Design review of the part built by this model. Coordinates are the model's own, in mm. A direction names the side the tool comes from. Coordinates: 2 decimals unless noted, no trailing zeros. Write each loop counter-clockwise with the first axis right and the second up, starting at its lowest first coordinate (ties: lowest second). Pieces come first, ordered by that corner, then holes.
Q1. Add section D-D, the plane x = -5.5. Give the boundary of the cut face in (y, z).
Q2. To check wall thickness, follow probe 1 along Y at (x, z) = (20, 3); probe 2 along X at (y, z) = (4, -53.5); probe 3 along Z at (x, y) = (36.5, 8). State the ranges of each line that lie inside material, in increasing order.
Q3. Add section C-C, the plane x = -16.5. Give the boundary of the cut face in (y, z).
Q4. Clearance check with flat-ended pins moving along their axes: pin 1 Ø2.5 at (x, y) = (-34.5, 29) entering from +Z; pin 2 Ø0.9 at (x, y) = (-35, 29) entering from -Z; pin 3 Ø12 at (x, z) = (-25.5, 26.5) entering from +Y. State where each tip first meets the part, or that it passes through.
Q5. The part is to be moulded in two halves that separate along X. For faces 1 (the face through (2, 0, 1)), 2 (the face through (38, 2, 73)), 3 (the face through (24.847, 12.86, 87.158)), say which applies: +X half, -X half, draft (parallel to the pull), parting line (faces both ways), or undercut.
Q6. Machinability: for faces 4 (the face through (-24.451, 12.86, 87.316)), 5 (the face through (-38, 9, -80.5)), 6 (the face through (-41.019, 17, -1)), 7 (the face through (38, 2, -73)), which of the approach directions +Z, -Z, +X, -X, +Y, -Y give a long, thin tool a straight path to every point of the face, cutting with its end or side? Answer none if there is none.
Q7. Add section B-B, the plane y = 15.5. Give the boundary of the cut face in (x, z).
Autodesk Inventor part; units mm, degrees
ref_plane "YZ Plane" through (0, 0, 0) normal (1, 0, 0) x (0, 1, 0)
ref_plane "XZ Plane" through (0, 0, 0) normal (0, 1, 0) x (-1, 0, 0)
ref_plane "XY Plane" through (0, 0, 0) normal (0, 0, 1) x (1, 0, 0)
sketch "Sketch1" plane through (0, 0, 0) normal (0, 1, 0) x (-1, 0, 0)
  line L0 (38, 68) -> (38, -68)
  line L1 (-38, -68) -> (-38, 68)
  line L2 (-38, 68) -> (38, -68) construction
  line L3 (38, 68) -> (-38, -68) construction
  line L4 (0, -68) -> (0, -80)
  arc A0 (-38, -68) -> (38, -68) centre (0, -13.8333) ccw
  arc A1 (38, 68) -> (-38, 68) centre (0, 13.8333) ccw
  line L5 (38, -68) -> (38, 68)
  line L6 (-38, 68) -> (-38, 53)
  line L7 (-38, -68) -> (-38, -53)
  line L8 (-38, -53) -> (-38, -34)
  line L9 (-38, 53) -> (-38, 34)
  line L10 (38, -68) -> (38, 68)
  line L11 (38, 68) -> (41, 68)
  line L12 (41, 68) -> (41, -68)
  line L13 (41, -68) -> (38, -68)
  line L14 (38, -68) -> (38, 68)
  line L15 (-38, 68) -> (-38, 53)
  line L16 (-38, 34) -> (-38, 53)
  line L17 (-38, -68) -> (-38, -53)
  line L18 (-38, -34) -> (-38, -53)
  line L19 (-38, 68) -> (-38, 52.5)
  line L20 (-38, 52.5) -> (-44, 52.5)
  line L21 (-44, 52.5) -> (-44, 33.5)
  line L22 (-44, 33.5) -> (-38, 33.5)
  line L23 (-38, 33.5) -> (-38, 52.5)
  line L24 (-38, 33.5) -> (-38, -33.5)
  line L25 (-38, -33.5) -> (-44, -33.5)
  line L26 (-44, -33.5) -> (-44, -52.5)
  line L27 (-44, -52.5) -> (-38, -52.5)
  line L28 (-38, -52.5) -> (-38, -33.5)
  point P0 (0, 0)
  dimension "d129" = 3
extrude "taban" add sketch "Sketch1" along normal blind 3
sketch "Sketch2" plane through (0, 3, 0) normal (0, 1, 0) x (1, 0, 0)
  line L0 (-41.0189, -68) -> (-38.0189, -68)
  line L1 (-38.0189, -68) -> (-38.0189, 68)
  line L2 (-38.0189, 68) -> (-41.0189, 68)
  line L3 (-41.0189, 68) -> (-41.0189, -68)
  point P0 (0, 0)
  dimension "d45" = 3
  dimension "d46" = 136
extrude "direk" add sketch "Sketch2" along normal blind 28
sketch "Sketch5" plane through (-38.0189, 3, 68) normal (1, 0, 0) x (0, 0, -1)
  line L0 (15.5, 28) -> (34.5, 28)
  line L1 (34.5, 28) -> (34.5, 25)
  line L2 (34.5, 25) -> (15.5, 25)
  line L3 (15.5, 25) -> (15.5, 28)
  line L4 (101.5, 28) -> (120.5, 28)
  line L5 (120.5, 28) -> (120.5, 25)
  line L6 (120.5, 25) -> (101.5, 25)
  line L7 (101.5, 25) -> (101.5, 28)
  point P0 (68, -3)
  point P1 (0, 28)
extrude "sikigecme" add sketch "Sketch5" along normal blind 7
sketch "Sketch6" plane through (0, 3, 0) normal (0, 1, 0) x (1, 0, 0)
  line L0 (-41, -68) -> (-38, -68)
  line L1 (-38, -68) -> (-38, -83)
  arc A0 (-38, -68) -> (38, -68) centre (0, -13.8333) ccw
  line L2 (38, -68) -> (38, -83)
  arc A1 (-38, -83) -> (38, -83) centre (0, -28.8333) ccw
  arc A2 (38, 68) -> (-38, 68) centre (0, 13.8333) ccw
  line L3 (-38, 68) -> (-38, 83)
  line L4 (38, 68) -> (38, 83)
  arc A3 (38, 83) -> (-38, 83) centre (0, 28.8333) ccw
  arc A4 (-38, -68) -> (38, -68) centre (0, -13.8333) ccw
  arc A5 (38, 68) -> (-38, 68) centre (0, 13.8333) ccw
  point P0 (0, 0)
  dimension "d66" = 15
  dimension "d67" = 15
  dimension "d99" = 15
  dimension "d100" = 15
extrude "fazlalik" add sketch "Sketch6" against normal blind 3
sketch "Sketch7" plane through (0, 3, 0) normal (0, 1, 0) x (1, 0, 0)
  arc A0 (-38, -83) -> (38, -83) centre (0, -28.8333) ccw
  line L0 (-38, -83) -> (-38, -80)
  line L1 (38, -83) -> (38, -80)
  arc A1 (-38, -80) -> (38, -80) centre (0, -25.8333) ccw
  arc A2 (-38, -83) -> (38, -83) centre (0, -28.8333) ccw
  arc A3 (38, 83) -> (-38, 83) centre (0, 28.8333) ccw
  line L2 (-38, 83) -> (-38, 80)
  line L3 (-38, 68) -> (-38, 83)
  line L4 (38, 52.5) -> (38, 83)
  line L5 (38, 83) -> (38, 80)
  arc A4 (38, 80) -> (-38, 80) centre (0, 25.8333) ccw
  arc A5 (38, 83) -> (-38, 83) centre (0, 28.8333) ccw
  point P0 (0, 0)
  point P1 (38, 53)
  point P2 (38, -34)
  dimension "d74" = 3
  dimension "d75" = 3
  dimension "d102" = 3
  dimension "d103" = 3
extrude "yandirek" add sketch "Sketch7" along normal blind 20
sketch "Sketch9" plane through (0, 3, 0) normal (0, 1, 0) x (1, 0, 0)
  arc A0 (-38, -83) -> (38, -83) centre (0, -28.8333) ccw
  line L0 (-10, -94.24) -> (-10, -91.24)
  arc A1 (-38, -80) -> (38, -80) centre (0, -25.8333) ccw
  line L1 (10, -94.24) -> (10, -91.24)
  arc A2 (-10, -94.24) -> (10, -94.24) centre (0, -28.8333) ccw
  arc A3 (-10, -91.24) -> (10, -91.24) centre (0, -25.8333) ccw
  arc A4 (38, 83) -> (-38, 83) centre (0, 28.8333) ccw
  line L2 (10.1599, 94.2153) -> (10, 91.24)
  arc A5 (38, 80) -> (-38, 80) centre (0, 25.8333) ccw
  line L3 (-10, 94.24) -> (-10, 91.24)
  arc A6 (10, 91.24) -> (-10, 91.24) centre (0, 25.8333) ccw
  arc A7 (10.1599, 94.2153) -> (-10, 94.24) centre (0, 28.8333) ccw
  point P0 (0, 0)
  point P1 (10, -91.24)
  point P2 (-10, 94.24)
extrude "yanbosluk" cut sketch "Sketch9" along normal blind 20
properties part number "VR_Telefon_Tutucu_3DPrint"
Here are the results:
1. outline: (0, -94.77) - (3, -94.77) - (3, 94.77) - (0, 94.77) - close
2. probe 1: y = 0 to 3
2. probe 2: x = -41.02 to -38.02
2. probe 3: z = -84.02 to -81.02, 81.02 to 84.02
3. outline: (0, -92.91) - (23, -92.91) - (23, -89.91) - (3, -89.91) - (3, 89.91) - (23, 89.91) - (23, 92.91) - (0, 92.91) - close
4. pin 1: stops at z = 52.5
4. pin 2: stops at z = -52.5
4. pin 3: stops at y = 3
5. face 1: draft
5. face 2: +X half
5. face 3: undercut
6. face 4: +Y
6. face 5: -Z, -X, +Y, -Y
6. face 6: +Z, -Z, -X, +Y, -Y
6. face 7: -Z, +X, +Y, -Y
7. outline: (-41.02, -68) - (-38.02, -68) - (-38.02, 68) - (-41.02, 68) - close; (-38, -83) arc R66.17 ccw to (-10, -94.24) - (-10, -91.24) arc R66.17 cw to (-38, -80) - close; (-38, 80) arc R66.17 cw to (-10, 91.24) - (-10, 94.24) arc R66.17 ccw to (-38, 83) - close; (10, -91.24) - (10.16, -94.22) arc R66.17 ccw to (38, -83) - (38, -80) arc R66.17 cw to start; (10, 91.24) arc R66.17 cw to (38, 80) - (38, 83) arc R66.17 ccw to (10, 94.24) - close
